from build123d import *

# Parameters (mm, degrees)
F0_R          = 15
F1_DEPTH      = 220
F1_DEPTH_BACK = 220
F3_DEPTH      = 10


with BuildPart() as f1:
    # F0 (on Right) → F1 (new body, two sides)
    with BuildSketch(Plane.YZ) as f1_sk:
        with BuildLine():
            Line((0, 100), (0, 0))
            Line((0, 0), (570, 0))
            Line((570, 0), (582.8065256566, 125.2091964617))
            ThreePointArc((582.8065256566, 125.2091964617), (563.9765046368, 175.2525352812), (512.6990361213, 190.4026730514))
            Line((512.6990361213, 190.4026730514), (0, 100))
        make_face()
        with Locations((475, 135)):
            Circle(F0_R, mode=Mode.SUBTRACT)
    extrude(amount=-F1_DEPTH)
    extrude(f1_sk.sketch, amount=F1_DEPTH_BACK)

    # F2 (on face) → F3 (join)
    with BuildSketch(Plane.YZ.offset(220)):
        with BuildLine():
            Line((44.4880730518, 137.4484157784), (44.4880730518, 107.8444475988))
            Line((44.4880730518, 107.8444475988), (74.4880730518, 113.13425702))
            Line((74.4880730518, 113.13425702), (74.4880730518, 142.7382251997))
            ThreePointArc((74.4880730518, 142.7382251997), (49.79055467, 195.090680183), (44.4880730518, 137.4484157784))
        make_face()
    extrude(amount=-F3_DEPTH)

    # F4: F1 across plane


with BuildPart() as f1_1:
    add(f1.part)
    add(f1.part.mirror(Plane.YZ))


solid = f1_1.part
Verification items for the finished model (mm, model axes). A direction names the side the tool comes from. Give positions to 0.01 mm unless a question says otherwise; leave off trailing zeros. Write each loop counter-clockwise with the first axis right and the second up, starting at its lowest first coordinate (ties: lowest second). Pieces come first, ordered by that corner, then holes. Notation, with made-up numbers: (65, 15.5) - (114, 15.5) arc R16 ccw to (114, 45.5) - close; hole circle Ø8 at (34.5, 61.25). An arc over 180 degrees is marked (long way). Answer as CSV lines item,"result". Start each with the question number.
1. Sectioned sample at C-C (y = 55). Record the boundary of the cut face in (x, z).
2. Sectioned sample at A-A (y = 475). Record the boundary of the cut face in (x, z).
3. Sectioned sample at D-D (z = 32). Record the boundary of the cut face in (x, y), then the cut area to 3 significant figures.
4. Thickness scan on line 1 (X direction, y = 58.5, z = 171.5); line 2 (Z direction, x = 32, y = 475); line 3 (Y direction, x = 56.5, z = 93). Record the ranges inside material, lowest first.
5. Set-up check for faces 4 (the face through (-210, 55, 152)), 5 (the face through (220, 287, 77)): record each of +Z, -Z, +X, -X, +Y, -Y from which the full face is reachable in a straight line by a thin tool's end or side.
6. Sectioned sample at B-B (x = -90). Record the boundary of the cut face in (y, z).
7. Draft check along Z on faces 1 (the face through (-3, 0, 51)), 2 (the face through (-215.07, 50.87, 195.26)), 3 (the face through (-3.08, 576.314, 61.728)). Enter one of: pulls with the +Z half, pulls with the -Z half, needs draft (parallel to the pull), parting line crosses it, or undercut.
8. Depth check by flat-ended pin: pin 1 (10 mm diameter, centred on x = 172.5, y = 76, fed in from +Z); pin 2 (11 mm diameter, centred on x = -213, z = 125.5, fed in from +Y); pin 3 (6 mm diameter, centred on x = -133, y = 514, fed in from +Z). Enter the tip coordinate at first touch or a pass-through.
Derived:
1,outline,"(-220, 0) - (220, 0) - (220, 195.55) - (210, 195.55) - (210, 109.7) - (-210, 109.7) - (-210, 195.55) - (-220, 195.55) - close"
2,outline,"(-220, 0) - (220, 0) - (220, 120) - (-220, 120) - close; (-220, 150) - (220, 150) - (220, 183.76) - (-220, 183.76) - close"
3,outline,"(-220, 0) - (220, 0) - (220, 573.27) - (-220, 573.27) - close"
3,area,"252,000 mm²"
4,line 1,"-220 to -210, 210 to 220"
4,line 2,"0 to 120, 150 to 183.76"
4,line 3,"0 to 579.51"
5,face 4,"+Z, -Y"
5,face 5,"+Z, -Z, +X, +Y, -Y"
6,outline,"(0, 0) - (570, 0) - (582.81, 125.21) arc R60 ccw to (512.7, 190.4) - (0, 100) - close; hole circle Ø30 at (475, 135)"
7,face 1,"needs draft"
7,face 2,"undercut"
7,face 3,"pulls with the -Z half"
8,pin 1,"z = 114.28"
8,pin 2,"y = 583.12"
8,pin 3,"z = 191"
